from build123d import *

# Parameters (mm, degrees)
F1_DEPTH = 38.1
F2_W     = 12.7
F2_H     = 6.35
F3_DEPTH = 12.7
F4_DEPTH = 12.7
F5_W     = 12.7
F5_H     = 6.35
F6_DEPTH = 12.7


with BuildPart() as f1:
    # F0 (on Front) → F1 (new body)
    with BuildSketch(Plane.XZ):
        Polygon((-43.0376454253, 49.6439802366), (-55.7376454253, 49.6439802366), (-55.7376454253, 17.8939802366), (-30.3376454253, 17.8939802366), (-30.3376454253, 30.5939802366), (-43.0376454253, 30.5939802366), align=None)
    extrude(amount=F1_DEPTH)

    # F2 (on face) → F3 (join)
    with BuildSketch(Plane.YZ.offset(-43.0376454253)):
        with Locations((-17.718813771, 46.4689802366)):
            Rectangle(F2_W, F2_H)
    extrude(amount=F3_DEPTH)

    # F4 (cut): a face of the model
    f4_faces = [f1.faces().sort_by_distance(p)[0] for p in [
        (-30.3376454253, -17.718813771, 46.4689802366),
    ]]
    extrude(f4_faces, amount=-F4_DEPTH, mode=Mode.SUBTRACT)

    # F5 (on face) → F6 (cut)
    with BuildSketch(Plane.YZ.offset(-43.0376454253)):
        with Locations((-19.05, 46.4689802366)):
            Rectangle(F5_W, F5_H)
    extrude(amount=-F6_DEPTH, mode=Mode.SUBTRACT)


solid = f1.part
CAD build for the part. Positions are in the model's coordinates, mm. A direction names the side the tool comes from. Give positions to 0.01 mm unless a question says otherwise; leave off trailing zeros. Write each loop counter-clockwise with the first axis right and the second up, starting at its lowest first coordinate (ties: lowest second). Pieces come first, ordered by that corner, then holes. Notation, with made-up numbers: (56, -4) -> (89, -4) arc R16 cw to (89, 3) -> close; hole circle Ø1 at (2.5, 40.25). An arc over 180 degrees is marked (long way). Return JSON: item names as keys, results as strings.
Item 1: Drill centre lines: probe 1 along Z at (x, y) = (-42.5, -30.5); probe 2 along X at (y, z) = (-29, 39); probe 3 along Z at (x, y) = (-45.5, -14). Where is each one in solid material? Low to high.
Answer below:
{"probe 1": "z = 17.89 to 30.59", "probe 2": "x = -55.74 to -43.04", "probe 3": "z = 17.89 to 43.29"}
Item 2: Band-saw the part on B-B (y = -17.5). List the corners of the cut face in (x, z).
Answer below:
{"outline": "(-55.74, 17.89) -> (-30.34, 17.89) -> (-30.34, 30.59) -> (-43.04, 30.59) -> (-43.04, 43.29) -> (-55.74, 43.29) -> close"}
Item 3: Band-saw the part on D-D (z = 31.5). List the corners of the cut face in (x, y), then the cut area to 3 significant figures.
Answer below:
{"outline": "(-55.74, -38.1) -> (-43.04, -38.1) -> (-43.04, 0) -> (-55.74, 0) -> close", "area": "484 mm2"}
Item 4: Band-saw the part on C-C (x = -47). List the corners of the cut face in (y, z).
Answer below:
{"outline": "(-38.1, 17.89) -> (0, 17.89) -> (0, 49.64) -> (-12.7, 49.64) -> (-12.7, 43.29) -> (-25.4, 43.29) -> (-25.4, 49.64) -> (-38.1, 49.64) -> close"}
Item 5: Two-plate mould, pull along Y, no slides. Class faces 4 (the flat face through (-49, -6, 49.644)), 5 (the flat face through (-49, -12.7, 46)), 6 (the flat face through (-46, 0, 30)): +Y half, -Y half, draft (parallel to the pull), parting line (faces both ways), or undercut.
Answer below:
{"face 4": "draft", "face 5": "undercut", "face 6": "+Y half"}
Item 6: Drop flat-ended pins along their axis: pin 1 (4 mm diameter, centred on y = -30.5, z = 42, fed in from +X); pin 2 (14 mm diameter, centred on x = -34, y = -15.5, fed in from +Z); pin 3 (5 mm diameter, centred on x = -38.5, z = 34, fed in from -Y); pin 4 (2 mm diameter, centred on x = -46.5, y = -15.5, fed in from +Z). Give the stop position or say it passes through.
Answer below:
{"pin 1": "stops at x = -43.04", "pin 2": "stops at z = 30.59", "pin 3": "passes through", "pin 4": "stops at z = 43.29"}
Item 7: Tool access for faces 1 (the flat face through (-49, -25.4, 46)), 2 (the flat face through (-43.038, -19, 40)), 3 (the flat face through (-55.738, -19, 34)): list every direction of +Z, -Z, +X, -X, +Y, -Y with a clear straight run to the whole face (end or side of a thin tool).
Answer below:
{"face 1": "+Z, +X, -X", "face 2": "+Z, +X, +Y, -Y", "face 3": "+Z, -Z, -X, +Y, -Y"}
Item 8: Band-saw the part on A-A (z = 45.5). List the corners of the cut face in (x, y).
Answer below:
{"outline": "(-55.74, -38.1) -> (-43.04, -38.1) -> (-43.04, -25.4) -> (-55.74, -25.4) -> close; (-55.74, -12.7) -> (-43.04, -12.7) -> (-43.04, 0) -> (-55.74, 0) -> close"}
